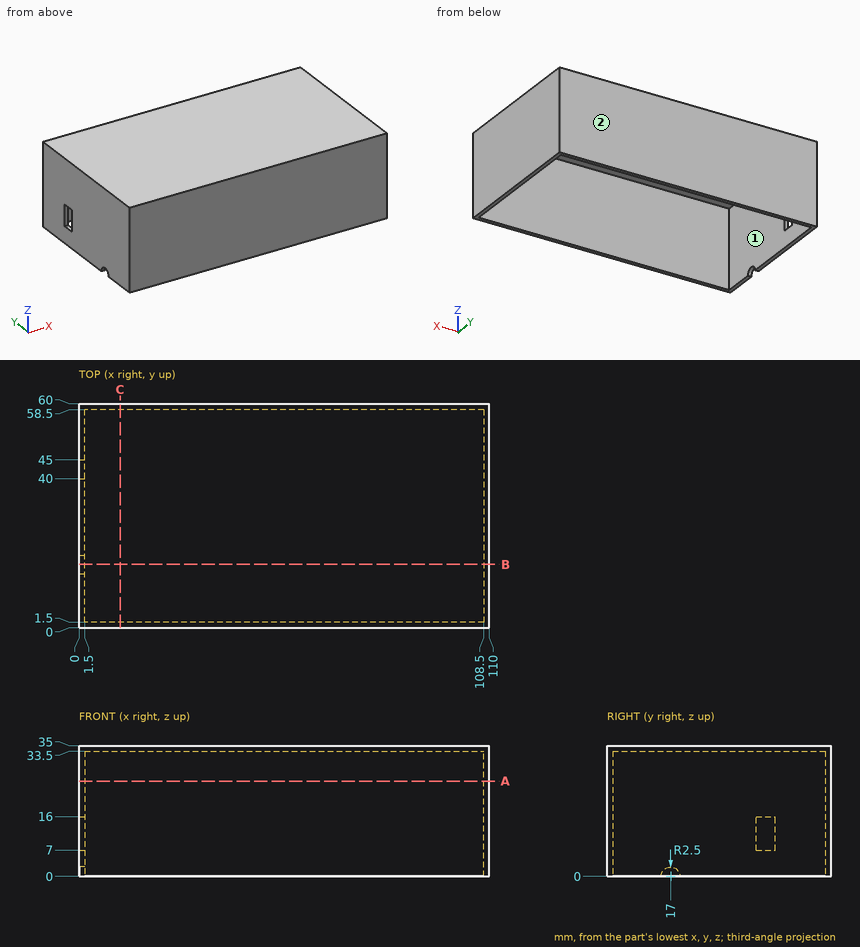
Geometry: see drawing. Coordinates: mm, zero at the bounding-box minimum. A direction names the side the tool comes from. Coordinates: 2 decimals unless noted, no trailing zeros. Order: outer loops, then holes, each group sorted by start corner. A loop starts at its lowest first (then second) coordinate and runs counter-clockwise, first axis right, second up. Notation, with made-up numbers: (20.25, 45) - (71.25, 45) arc R19 ccw to (71.25, 77) - close; hole circle Ø2 at (52.25, 82). An arc over 180 degrees is marked (long way). Write each question's results on one line, items separated by ' | '.
1) Pin query (flat end, axial travel): pin 1 (17 mm diameter, centred on y = 31.5, z = 11.5, fed in from -X). Return the tip coordinate at first contact, or that it passes through.
Results list:
pin 1: x = 0
2) Section B-B, the plane y = 17. Return loops of the section in (x, z).
Results list:
outline: (0, 2.5) - (1.5, 2.5) - (1.5, 33.5) - (108.5, 33.5) - (108.5, 0) - (110, 0) - (110, 35) - (0, 35) - close
3) Set-up query: the marked faces 1 and 2. Return all of +Z, -Z, +X, -X, +Y, -Y with unobstructed straight access to the full face (end or side cutting, diameter ignored); none if empty.
Results list:
face 1: -Z | face 2: +Z, -Z, +X, -X, +Y
4) Section A-A, the plane z = 25.5. Return loops of the section in (x, y), plus the area to 3 significant figures.
Results list:
outline: (0, 0) - (110, 0) - (110, 60) - (0, 60) - close; hole (1.5, 1.5) - (108.5, 1.5) - (108.5, 58.5) - (1.5, 58.5) - close | area: 501 mm^2
5) Section C-C, the plane x = 11. Return loops of the section in (y, z), plus the area to 4 significant figures.
Results list:
outline: (0, 0) - (1.5, 0) - (1.5, 33.5) - (58.5, 33.5) - (58.5, 0) - (60, 0) - (60, 35) - (0, 35) - close | area: 190.5 mm^2
6) Line query: line 1 (X direction, y = 53, z = 27.5); line 2 (Y direction, x = 29, z = 17); line 3 (Z direction, x = 66, y = 38.5). Output: solid intervals per line, ascending. Write a range as from..to.
Results list:
line 1: 0..1.5, 108.5..110 | line 2: 0..1.5, 58.5..60 | line 3: 33.5..35
